from build123d import *

# Parameters (mm, degrees)
F0_R     = 11
F1_DEPTH = 1
F0_R_2   = 12.2
F2_DEPTH = 10
F3_R     = 11.6
F3_R_2   = 11
F4_DEPTH = 1
F6_DEPTH = 8


with BuildPart() as f1:
    # F0 (on Top) → F1 (new body)
    with BuildSketch(Plane.XY):
        with Locations((-31.5797176751, 0)):
            Circle(F0_R)
    extrude(amount=F1_DEPTH)

    # F0 (on Top) → F2 (join)
    with BuildSketch(Plane.XY):
        with Locations((-31.5797176751, 0)):
            Circle(F0_R_2)
        with Locations((-31.5797176751, 0)):
            Circle(F0_R, mode=Mode.SUBTRACT)
    extrude(amount=F2_DEPTH)

    # F3 (on face) → F4 (cut)
    with BuildSketch(Plane.XY.offset(10)):
        with Locations((-31.5797176751, 0)):
            Circle(F3_R)
        with Locations((-31.5797176751, 0)):
            Circle(F3_R_2, mode=Mode.SUBTRACT)
    extrude(amount=-F4_DEPTH, mode=Mode.SUBTRACT)

    # F5 (on face) → F6 (cut)
    with BuildSketch(Plane.XY.offset(10)):
        with BuildLine():
            ThreePointArc((-19.3797176751, 0), (-19.4737308076, 1.511648757), (-19.7543212758, 3))
            Line((-19.7543212758, 3), (-20.3743618128, 3))
            ThreePointArc((-20.3743618128, 3), (-20.0788018854, 1.5129229983), (-19.9797176751, 0))
            ThreePointArc((-19.9797176751, 0), (-20.0788018854, -1.5129229983), (-20.3743618128, -3))
            Line((-20.3743618128, -3), (-19.7543212758, -3))
            ThreePointArc((-19.7543212758, -3), (-19.4737308076, -1.511648757), (-19.3797176751, 0))
        make_face()
        with BuildLine():
            Line((-20.3743618128, 3), (-42.7850735373, 3))
            ThreePointArc((-42.7850735373, 3), (-43.1797176751, 0), (-42.7850735373, -3))
            Line((-42.7850735373, -3), (-20.3743618128, -3))
            ThreePointArc((-20.3743618128, -3), (-20.0788018854, -1.5129229983), (-19.9797176751, 0))
            ThreePointArc((-19.9797176751, 0), (-20.0788018854, 1.5129229983), (-20.3743618128, 3))
        make_face()
        with BuildLine():
            Line((-42.7850735373, 3), (-43.4051140743, 3))
            ThreePointArc((-43.4051140743, 3), (-43.7797176751, 0), (-43.4051140743, -3))
            Line((-43.4051140743, -3), (-42.7850735373, -3))
            ThreePointArc((-42.7850735373, -3), (-43.1797176751, 0), (-42.7850735373, 3))
        make_face()
    extrude(amount=-F6_DEPTH, mode=Mode.SUBTRACT)


solid = f1.part
Work out the finished part from the listing and answer in its coordinate system (mm). A direction names the side the tool comes from. Give positions to 0.01 mm unless a question says otherwise; leave off trailing zeros. Order: outer loops, then holes, each group sorted by start corner. A loop starts at its lowest first (then second) coordinate and runs counter-clockwise, first axis right, second up. Notation, with made-up numbers: (29.25, 1) -> (52.25, 1) arc R24 cw to (52.25, 32) -> close; hole circle Ø9 at (59, 69.5). An arc over 180 degrees is marked (long way). Answer as a JSON object with one key per item and string values. Group by question number.
1. Section B-B on y = 0 is taken. Determine the outline of the cut face in (x, z), plus the area to 3 significant figures.
2. Consider line 1 along Y through (x, z) = (-31.5, 9.25); line 2 along Z through (x, y) = (-39, -3.75); line 3 along X through (y, z) = (3.75, 5.5). Determine where each line is inside the solid, lowest interval first. Write a range as [from, to].
3. Section D-D on x = -22 is taken. Determine the outline of the cut face in (y, z), plus the area to 3 significant figures.
4. The mould has two halves that part along Y. Classify faces 1 (the cylindrical face through (-21.419, -4.213, 4.944)), 2 (the cylindrical face through (-19.94, 3.66, 4.93)), 3 (the flat face through (-32, 0, 0)): released by +Y, released by -Y, zero draft, split by the parting line, or undercut.
5. Section A-A on z = 8 is taken. Determine the outline of the cut face in (x, y).
6. Section C-C on x = -36.25 is taken. Determine the outline of the cut face in (y, z).
7. A tool of negligible diameter and unlimited length cuts with its end or side. For faces 4 (the flat face through (-32, 0, 1)), 5 (the flat face through (-20, -3, 6)), 6 (the flat face through (-32, -12, 10)), from which of +Z, -Z, +X, -X, +Y, -Y can it reach the whole face along a straight path? Write none if from no direction.
8. Flat-ended cylindrical pins translate along their axes: pin 1 Ø0.6 at (x, z) = (-20.5, 4) entering from +Y; pin 2 Ø1.4 at (x, z) = (-43, 4) entering from +Y; pin 3 Ø4 at (x, z) = (-34.5, 1) entering from +Y. Find the tip coordinate at first contact, or state that the pin passes through.
Result sheet:
{
 "1": {"outline": "(-43.78, 0) -> (-19.38, 0) -> (-19.38, 2) -> (-20.58, 2) -> (-20.58, 1) -> (-42.58, 1) -> (-42.58, 2) -> (-43.78, 2) -> close", "area": "26.8 mm^2"},
 "2": {"line 1": "y = [-12.2, -11.6], [11.6, 12.2]", "line 2": "z = [0, 1]", "line 3": "x = [-43.19, -41.92], [-21.24, -19.97]"},
 "3": {"outline": "(-7.55, 0) -> (7.55, 0) -> (7.55, 10) -> (6.54, 10) -> (6.54, 9) -> (5.41, 9) -> (5.41, 1) -> (-5.41, 1) -> (-5.41, 9) -> (-6.54, 9) -> (-6.54, 10) -> (-7.55, 10) -> close", "area": "51.5 mm^2"},
 "4": {"face 1": "undercut", "face 2": "split by the parting line", "face 3": "zero draft"},
 "5": {"outline": "(-43.41, -3) arc R12.2 ccw to (-19.75, -3) -> (-21, -3) arc R11 cw to (-42.16, -3) -> close; (-43.41, 3) -> (-42.16, 3) arc R11 cw to (-21, 3) -> (-19.75, 3) arc R12.2 ccw to start"},
 "6": {"outline": "(-11.27, 0) -> (11.27, 0) -> (11.27, 10) -> (10.62, 10) -> (10.62, 9) -> (9.96, 9) -> (9.96, 1) -> (-9.96, 1) -> (-9.96, 9) -> (-10.62, 9) -> (-10.62, 10) -> (-11.27, 10) -> close"},
 "7": {"face 4": "+Z", "face 5": "+Z, +X, -X", "face 6": "+Z, +X, -X, +Y, -Y"},
 "8": {"pin 1": "stops at y = 5.71", "pin 2": "stops at y = 5.82", "pin 3": "stops at y = 12.17"}
}
